Geometry: final body of the model. Coordinates: model frame, mm. A direction names the side the tool comes from. Round coordinates to 2 decimals unless told otherwise and drop trailing zeros. Loops run counter-clockwise (first coordinate to the right, second up) from the corner with the lowest first, then second, coordinate; pieces in that order, holes last. Notation, with made-up numbers: (28.25, 82) - (86.25, 82) arc R10 cw to (86.25, 94) - close; hole circle Ø11 at (87.25, 60). An arc over 180 degrees is marked (long way). Use CSV: the item, a comma, the result in double quotes.
from build123d import *

# Parameters (mm, degrees)
SKETCH1_R           = 1.1
SKETCH1_R_2         = 1.6
BOSS_EXTRUDE1_DEPTH = 3


with BuildPart() as part:
    # Sketch1 → Boss-Extrude1 (new body)
    with BuildSketch(Plane(origin=(0, 0, 0), x_dir=(1, 0, 0), z_dir=(0, 1, 0))):
        with BuildLine():
            Line((-28, 25), (-28, -25))
            Line((-28, -25), (-43.301270189, -25))
            ThreePointArc((-43.301270189, -25), (0, -50), (43.301270189, -25))
            Line((43.301270189, -25), (28, -25))
            Line((28, -25), (28, 25))
            Line((28, 25), (43.301270189, 25))
            ThreePointArc((43.301270189, 25), (0, 50), (-43.301270189, 25))
            Line((-43.301270189, 25), (-28, 25))
        make_face()
        with Locations((-11, 9)):
            Circle(SKETCH1_R, mode=Mode.SUBTRACT)
        with Locations((-7.5, 40)):
            Circle(SKETCH1_R, mode=Mode.SUBTRACT)
        with Locations((-7.5, -40)):
            Circle(SKETCH1_R, mode=Mode.SUBTRACT)
        with Locations((-11, -9)):
            Circle(SKETCH1_R, mode=Mode.SUBTRACT)
        with Locations((7.5, -40)):
            Circle(SKETCH1_R, mode=Mode.SUBTRACT)
        with Locations((7.5, 40)):
            Circle(SKETCH1_R, mode=Mode.SUBTRACT)
        with Locations((11, 9)):
            Circle(SKETCH1_R, mode=Mode.SUBTRACT)
        with Locations((11, -9)):
            Circle(SKETCH1_R, mode=Mode.SUBTRACT)
        with Locations((-35, 30)):
            Circle(SKETCH1_R_2, mode=Mode.SUBTRACT)
        with Locations((-35, -30)):
            Circle(SKETCH1_R_2, mode=Mode.SUBTRACT)
        with Locations((35, 30)):
            Circle(SKETCH1_R_2, mode=Mode.SUBTRACT)
        with Locations((35, -30)):
            Circle(SKETCH1_R_2, mode=Mode.SUBTRACT)
    extrude(amount=BOSS_EXTRUDE1_DEPTH)


solid = part.part
Item 1: Section A-A on z = -9. Return the cut outline in (x, y), plus the area to 3 significant figures.
Final values:
outline,"(-28, 0) - (-12.1, 0) - (-12.1, 3) - (-28, 3) - close; (-9.9, 0) - (9.9, 0) - (9.9, 3) - (-9.9, 3) - close; (12.1, 0) - (28, 0) - (28, 3) - (12.1, 3) - close"
area,"155 mm²"
Item 2: Pin query (flat end, axial travel): P1, Ø0.9, axis at x = 35, y = 2, coming from the -Z side; P2, Ø1.5, axis at x = -35.5, y = 1, coming from the +Z side; P3, Ø1.5, axis at y = 1, z = 3.5, coming from the +X side. Return the tip coordinate at first contact, or that it passes through.
Final values:
P1,"stops at z = -36.14"
P2,"stops at z = 35.95"
P3,"stops at x = 28"
Item 3: Section D-D on x = 7.5. Return the cut outline in (y, z), plus the area to 3 significant figures.
Final values:
outline,"(0, -49.43) - (3, -49.43) - (3, -41.1) - (0, -41.1) - close; (0, -38.9) - (3, -38.9) - (3, 38.9) - (0, 38.9) - close; (0, 41.1) - (3, 41.1) - (3, 49.43) - (0, 49.43) - close"
area,"283 mm²"
Item 4: Reachability of faces 4 (the flat face through (-36, 1, 25)), 5 (the flat face through (-1, 0, -1)), 6 (the flat face through (28, 1, 0)) from +Z, -Z, +X, -X, +Y, -Y: full face, straight path, thin tool, end or side. Return the list, or none.
Final values:
face 4,"-X, +Y, -Y"
face 5,"+Z, -Z, +X, -X, -Y"
face 6,"+X, +Y, -Y"
Item 5: Section C-C on x = 35. Return the cut outline in (y, z).
Final values:
outline,"(0, -35.71) - (3, -35.71) - (3, -31.6) - (0, -31.6) - close; (0, -28.4) - (3, -28.4) - (3, -25) - (0, -25) - close; (0, 25) - (3, 25) - (3, 28.4) - (0, 28.4) - close; (0, 31.6) - (3, 31.6) - (3, 35.71) - (0, 35.71) - close"
Item 6: Section B-B on y = 1.15. Give the number of separate pieces and of enclosed holes in the cut face, plus the area to 3 significant figures.
Final values:
separate pieces,"1"
enclosed holes,"12"
area,"5,810 mm²"
Item 7: Material intervals for line 1 (X direction, y = 2.6, z = -30); line 2 (Z direction, x = -11, y = 1.5) (3 decimals); line 3 (X direction, y = 1.75, z = 9), sorted ascending.
Final values:
line 1,"x = -40 to -36.6, -33.4 to 33.4, 36.6 to 40"
line 2,"z = -48.775 to -10.1, -7.9 to 7.9, 10.1 to 48.775"
line 3,"x = -28 to -12.1, -9.9 to 9.9, 12.1 to 28"
Item 8: Mould query, pull axis X, two halves, no side actions, for faces 1 (the cylindrical face through (33.82, 1.48, -31.08)), 2 (the cylindrical face through (0.733, 1.479, -49.995)), 3 (the flat face through (36, 1, -25)). Classes: released by +X, released by -X, zero draft, split by the parting line, or undercut.
Final values:
face 1,"undercut"
face 2,"split by the parting line"
face 3,"zero draft"
